Autodesk Inventor part; units mm, degrees
ref_plane "YZ Plane" through (0, 0, 0) normal (1, 0, 0) x (0, 1, 0)
ref_plane "XZ Plane" through (0, 0, 0) normal (0, 1, 0) x (-1, 0, 0)
ref_plane "XY Plane" through (0, 0, 0) normal (0, 0, 1) x (1, 0, 0)
sketch "Sketch1" plane through (0, 0, 0) normal (0, 0, 1) x (1, 0, 0)
  line L0 (0, 0) -> (3.175, 0)
  line L1 (3.175, 0) -> (3.175, 25.4)
  line L2 (3.175, 25.4) -> (0, 25.4)
  line L3 (0, 25.4) -> (0, 0)
  line L4 (0, 0) -> (25.4, 0)
  line L5 (25.4, 0) -> (25.4, 3.175)
  line L6 (25.4, 3.175) -> (0, 3.175)
  line L7 (0, 3.175) -> (0, 0)
  dimension "d0" = 3.175
  dimension "d1" = 25.4
  dimension "d2" = 25.4
  dimension "d3" = 3.175
extrude "Extrusion1" add sketch "Sketch1" along normal blind 50.8
sketch "Sketch2" plane through (3.175, 3.175, 0) normal (0, 1, 0) x (1, 0, 0)
  line L0 (-3.175, 0) -> (-3.175, -50.8) construction
  line L1 (-3.175, 0) -> (9.525, 0) construction
  line L2 (22.225, 0) -> (0, 0) construction
  line L3 (9.525, 0) -> (9.525, -25.4) construction
  circle A0 centre (9.525, -25.4) radius 1.9844
  dimension "d6" = 12.7
  dimension "d7" = 25.4
  dimension "d8" = 3.9688
extrude "Extrusion2" cut sketch "Sketch2" against normal blind 50.8
properties part number "1x1 L brackets 2in"
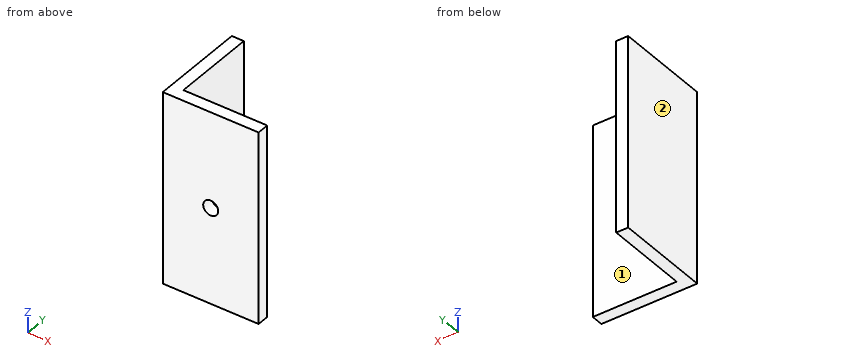
Can you work these out from the model? Positions are in its coordinate system, mm. Face numbers are marked on the shaded views. A direction names the side the tool comes from. Coordinates: 2 decimals unless noted, no trailing zeros. Write each loop counter-clockwise with the first axis right and the second up, starting at its lowest first coordinate (ties: lowest second). Pieces come first, ordered by that corner, then holes.
Q1. Which directions (+Z, -Z, +X, -X, +Y, -Y) give clear straight access to the entire face, cutting with the end or side of a thin tool? Please do the marked faces 1 and 2.
Results found:
face 1: +Z, -Z, +X, +Y
face 2: +Z, -Z, -X, +Y, -Y
Q2. Imagine slicing it at A-A, the plane x = 12.7. List the corners of the cut face in (y, z) for me (3 decimals), plus the area to 3 significant figures.
Results found:
outline: (0, 0) - (3.175, 0) - (3.175, 23.416) - (0, 23.416) - close; (0, 27.384) - (3.175, 27.384) - (3.175, 50.8) - (0, 50.8) - close
area: 149 mm2
Q3. For P1, Ø6.5, axis at y = 15, z = 32, coming from the +X side (3 decimals); P2, Ø11, axis at x = 17.5, z = 23, coming from the +Y side (3 decimals), each with a flat end and sliding along its axis, tell me the tip position at first contact or that it passes through.
Results found:
P1: stops at x = 3.175
P2: stops at y = 3.175
Q4. Imagine slicing it at D-D, the plane y = 7. List the corners of the cut face in (x, z) for me (3 decimals).
Results found:
outline: (0, 0) - (3.175, 0) - (3.175, 50.8) - (0, 50.8) - close
Q5. Imagine slicing it at C-C, the plane z = 34.5. List the corners of the cut face in (x, y) for me (3 decimals).
Results found:
outline: (0, 0) - (25.4, 0) - (25.4, 3.175) - (3.175, 3.175) - (3.175, 25.4) - (0, 25.4) - close
Q6. Please list where these lines run through material, in increasing order: L1, parallel to X at y = 1.65, z = 25.4; L2, parallel to Z at x = 12.7, y = 0.9; L3, parallel to Y at x = 8.5, z = 5 (3 decimals).
Results found:
L1: x = 0 to 10.72, 14.68 to 25.4
L2: z = 0 to 23.42, 27.38 to 50.8
L3: y = 0 to 3.175
Q7. Imagine slicing it at B-B, the plane z = 25.4. List the corners of the cut face in (x, y) for me (3 decimals), plus the area to 3 significant figures.
Results found:
outline: (0, 0) - (10.716, 0) - (10.716, 3.175) - (3.175, 3.175) - (3.175, 25.4) - (0, 25.4) - close; (14.684, 0) - (25.4, 0) - (25.4, 3.175) - (14.684, 3.175) - close
area: 139 mm2
